from build123d import *

# Parameters (mm, degrees)
SKETCH1_W           = 20
SKETCH1_H           = 22
SKETCH1_W_2         = 9
SKETCH1_H_2         = 3.65
BOSS_EXTRUDE1_DEPTH = 4
SKETCH2_W           = 10
SKETCH2_H           = 8
BOSS_EXTRUDE3_DEPTH = 4
SKETCH3_W           = 4.5
SKETCH3_H           = 3
CUT_EXTRUDE1_DEPTH  = 24.173260453
CHAMFER1_SIZE       = 0.5


with BuildPart() as part:
    # Sketch1 → Boss-Extrude1 (new body)
    with BuildSketch(Plane(origin=(0, 0, 0), x_dir=(1, 0, 0), z_dir=(0, 1, 0))):
        Rectangle(SKETCH1_W, SKETCH1_H)
        Rectangle(SKETCH1_W_2, SKETCH1_H_2, mode=Mode.SUBTRACT)
    extrude(amount=BOSS_EXTRUDE1_DEPTH)

    # Sketch2 → Boss-Extrude3 (add)
    with BuildSketch(Plane(origin=(0, 0, 0), x_dir=(1, 0, 0), z_dir=(0, 1, 0))):
        with Locations((15, 0)):
            Rectangle(SKETCH2_W, SKETCH2_H)
    extrude(amount=BOSS_EXTRUDE3_DEPTH)

    # Sketch3 → Cut-Extrude1 (cut, through all)
    with BuildSketch(Plane(origin=(0, 0, 0), x_dir=(1, 0, 0), z_dir=(0, 1, 0))):
        with Locations((14.75, 2.5)):
            Rectangle(SKETCH3_W, SKETCH3_H)
    extrude(amount=CUT_EXTRUDE1_DEPTH, mode=Mode.SUBTRACT)

    # Chamfer1
    chamfer1_edges = [part.edges().sort_by_distance(p)[0] for p in [
        (4.5, 0, 0),
        (0, 0, -1.825),
        (-4.5, 0, 0),
        (0, 0, 1.825),
        (10, 0, -7.5),
        (15, 0, 4),
        (20, 0, 0),
        (18.5, 0, -4),
        (11.25, 0, -4),
        (12.5, 0, -2.5),
        (14.75, 0, -1),
        (17, 0, -2.5),
        (0, 0, -11),
        (10, 0, 7.5),
        (0, 0, 11),
        (-10, 0, 0),
    ]]
    chamfer(chamfer1_edges, length=CHAMFER1_SIZE)


solid = part.part
Design review of the part built by this model. Coordinates are the model's own, in mm. A direction names the side the tool comes from. Give positions to 0.01 mm unless a question says otherwise; leave off trailing zeros. Loops run counter-clockwise (first coordinate to the right, second up) from the corner with the lowest first, then second, coordinate; pieces in that order, holes last. Notation, with made-up numbers: M 70.5,-27.5 L 118.5,-27.5 A16 ccw 118.5,-13.5 Z; hole C -10,88.5 d7. An arc over 180 degrees is marked long. One line per question, with ' | ' between items. Start each with the question number.
1. Insertion check: P1, Ø0.9, axis at x = 18, y = 1.5, coming from the -Z side; P2, Ø1.8, axis at y = 2.5, z = 7, coming from the +X side; P3, Ø1, axis at x = 14.5, y = 2, coming from the -Z side. Each pin has a flat end and moves straight along its axis. Give the tip position at first contact, or say it passes through.
2. To check wall thickness, follow L1, parallel to X at y = 0.8, z = -1.5; L2, parallel to Z at x = 4.25, y = 1.25 (3 decimals); L3, parallel to Z at x = -2, y = 0.35 (3 decimals). State the ranges of each line that lie inside material, in increasing order.
3. The part is to be moulded in two halves that separate along Z. For faces 1 (the face through (0, 2, -11)), 2 (the face through (0, 2, 1.825)), 3 (the face through (0, 2, 11)), say which applies: released by +Z, released by -Z, zero draft, split by the parting line, or undercut.
4. Add section B-B (y = 2.6). Write out the cut boundary in (x, z) (3 decimals), plus the area to 3 significant figures.
5. Add section D-D (x = 18). Write out the cut boundary in (y, z).
6. Add section C-C (x = 1). Write out the cut boundary in (y, z) (3 decimals), plus the area to 3 significant figures.
7. Add section A-A (z = 1.25). Write out the cut boundary in (x, y).
8. For faces 4 (the face through (15, 2, 4)), 5 (the face through (10, 2, -7)), 6 (the face through (17, 2, -2)), 7 (the face through (-4.5, 2, 0)), list the 3-axis set-ups (+Z, -Z, +X, -X, +Y, -Y) from which the entire face can be reached by the end or side of a thin tool; tool diameter is ignored.
Worked out:
1) P1: stops at z = -4 | P2: stops at x = 10 | P3: stops at z = -1
2) L1: x = -10 to -4.5, 4.5 to 12.5, 17 to 20 | L2: z = -11 to -1.825, 1.825 to 11 | L3: z = -10.85 to -1.975, 1.975 to 10.85
3) face 1: released by -Z | face 2: undercut | face 3: released by +Z
4) outline: M -10,-11 L 10,-11 L 10,-4 L 12.5,-4 L 12.5,-1 L 17,-1 L 17,-4 L 20,-4 L 20,4 L 10,4 L 10,11 L -10,11 Z; hole M -4.5,-1.825 L 4.5,-1.825 L 4.5,1.825 L -4.5,1.825 Z | area: 474 mm²
5) outline: M 0,-3.5 L 0.5,-4 L 4,-4 L 4,4 L 0.5,4 L 0,3.5 Z
6) outline: M 0,-10.5 L 0.5,-11 L 4,-11 L 4,-1.825 L 0.5,-1.825 L 0,-2.325 Z; M 0,2.325 L 0.5,1.825 L 4,1.825 L 4,11 L 0.5,11 L 0,10.5 Z | area: 72.9 mm²
7) outline: M -10,0.5 L -9.5,0 L -5,0 L -4.5,0.5 L -4.5,4 L -10,4 Z; M 4.5,0.5 L 5,0 L 19.5,0 L 20,0.5 L 20,4 L 4.5,4 Z
8) face 4: +Z, +X, +Y, -Y | face 5: -Z, +X, +Y, -Y | face 6: -Z, +Y, -Y | face 7: +Y, -Y
